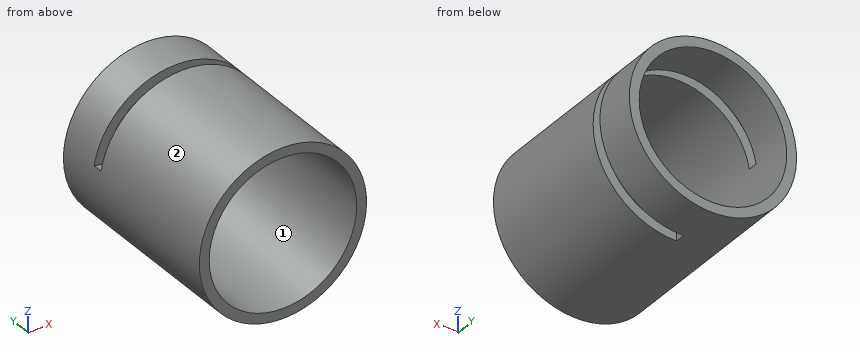
from build123d import *

# Parameters (mm, degrees)
SKETCH_1_R          = 25.5
SKETCH_1_R_2        = 22.5
EXTRUDE_1_DEPTH     = 60
SKETCH_2_W          = 46.809184836
SKETCH_2_H          = 3
CUT_REVOLVE_1_ANGLE = 260


with BuildPart() as part:
    # Sketch 1 → Extrude 1 (new body)
    with BuildSketch(Plane(origin=(0, 0, 0), x_dir=(1, 0, 0), z_dir=(0, 1, 0))):
        with Locations(Location((0, 0, 0), (0, 0, 270))):
            Circle(SKETCH_1_R)
        with Locations(Location((0, 0, 0), (0, 0, 270))):
            Circle(SKETCH_1_R_2, mode=Mode.SUBTRACT)
    extrude(amount=EXTRUDE_1_DEPTH)

    # Sketch 2 → Cut-Revolve 1 (revolve, cut)
    with BuildSketch(Plane(origin=(0, 0, 0), x_dir=(0, 0, -1), z_dir=(1, 0, 0))):
        with Locations((23.404592418, 45.5)):
            Rectangle(SKETCH_2_W, SKETCH_2_H)
    revolve(axis=Axis((0, 60.338123586, 0), (0, -1, 0)), revolution_arc=CUT_REVOLVE_1_ANGLE, mode=Mode.SUBTRACT)


solid = part.part
Read the model definition and answer for the solid it produces. Units are mm, in the model's axes. Face numbers are marked on the shaded views. Give positions to 0.01 mm unless a question says otherwise; leave off trailing zeros. Write each loop counter-clockwise with the first axis right and the second up, starting at its lowest first coordinate (ties: lowest second). Pieces come first, ordered by that corner, then holes. Notation, with made-up numbers: (64.25, -21) - (100.25, -21) arc R28 cw to (100.25, 7) - close; hole circle Ø6 at (15, 62.5). An arc over 180 degrees is marked (long way). Use CSV: the item, a comma, the result in double quotes. Start each with the question number.
Item 1: The part is cut by section A-A, the plane z = 0. Give the vertices of the cut face in (x, y), and give its area (3 significant figures).
Item 2: The part is cut by section D-D, the plane z = 9. Give the vertices of the cut face in (x, y).
Item 3: Flat-ended cylindrical pins translate along their axes: P1, Ø8, axis at y = 32, z = -6, coming from the +X side; P2, Ø10, axis at y = 41, z = -16, coming from the -X side; P3, Ø10, axis at x = -9, y = 42.5, coming from the -Z side. Find the tip coordinate at first contact, or state that the pin passes through.
Item 4: The part is cut by section B-B, the plane x = 15. Give the vertices of the cut face in (y, z), and give its area (3 significant figures).
Item 5: Consider line 1 (X direction, y = 41.5, z = 0); line 2 (X direction, y = 29, z = -9.5). Determine where each line is inside the solid, lowest interval first.
Item 6: The mould has two halves that part along X. Classify the marked faces 1 and 2: pulls with the +X half, pulls with the -X half, needs draft (parallel to the pull), parting line crosses it, or undercut.
Item 7: The part is cut by section C-C, the plane x = -20. Give the vertices of the cut face in (y, z), and give its area (3 significant figures).
Taken from the geometry:
1,outline,"(-25.5, 0) - (-22.5, 0) - (-22.5, 60) - (-25.5, 60) - close; (22.5, 0) - (25.5, 0) - (25.5, 44) - (22.5, 44) - close; (22.5, 47) - (25.5, 47) - (25.5, 60) - (22.5, 60) - close"
1,area,"351 mm2"
2,outline,"(-23.86, 0) - (-20.62, 0) - (-20.62, 44) - (-23.86, 44) - close; (-23.86, 47) - (-20.62, 47) - (-20.62, 60) - (-23.86, 60) - close; (20.62, 0) - (23.86, 0) - (23.86, 44) - (20.62, 44) - close; (20.62, 47) - (23.86, 47) - (23.86, 60) - (20.62, 60) - close"
3,P1,"x = 25.42"
3,P2,"x = -23.01"
3,P3,"z = -25.18"
4,outline,"(0, -20.62) - (44, -20.62) - (44, -16.77) - (0, -16.77) - close; (0, 16.77) - (44, 16.77) - (44, 20.62) - (0, 20.62) - close; (47, -20.62) - (60, -20.62) - (60, -16.77) - (47, -16.77) - close; (47, 16.77) - (60, 16.77) - (60, 20.62) - (47, 20.62) - close"
4,area,"439 mm2"
5,line 1,"-25.5 to -22.5, 22.5 to 25.5"
5,line 2,"-23.66 to -20.4, 20.4 to 23.66"
6,face 1,"undercut"
6,face 2,"parting line crosses it"
7,outline,"(0, -15.82) - (60, -15.82) - (60, -10.31) - (0, -10.31) - close; (0, 10.31) - (44, 10.31) - (44, 15.82) - (0, 15.82) - close; (47, 10.31) - (60, 10.31) - (60, 15.82) - (47, 15.82) - close"
7,area,"645 mm2"
